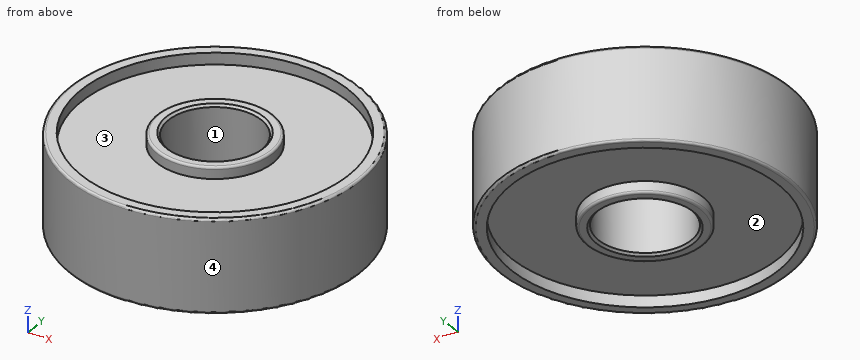
from build123d import *

# Parameters (mm, degrees)
F0_R     = 12.5
F1_DEPTH = 8
F2_R     = 4
F3_DEPTH = 8.001
F2_R_2   = 11.5
F2_R_3   = 5
F4_DEPTH = 1
F5_R     = 11.5
F5_R_2   = 5
F6_DEPTH = 1
F7_R     = 0.2
F8_SIZE  = 0.2


with BuildPart() as f1:
    # F0 (on Top) → F1 (new body)
    with BuildSketch(Plane.XY):
        Circle(F0_R)
    extrude(amount=F1_DEPTH)

    # F2 (on face) → F3 (cut, through all)
    with BuildSketch(Plane.XY.offset(8)):
        Circle(F2_R)
    extrude(amount=-F3_DEPTH, mode=Mode.SUBTRACT)

    # F2 (on face) → F4 (cut)
    with BuildSketch(Plane.XY.offset(8)):
        Circle(F2_R_2)
        Circle(F2_R_3, mode=Mode.SUBTRACT)
    extrude(amount=-F4_DEPTH, mode=Mode.SUBTRACT)

    # F5 (on face) → F6 (cut)
    with BuildSketch(Plane(origin=(0, 0, 0), x_dir=(1, 0, 0), z_dir=(0, 0, -1))):
        Circle(F5_R)
        Circle(F5_R_2, mode=Mode.SUBTRACT)
    extrude(amount=-F6_DEPTH, mode=Mode.SUBTRACT)

    # F7
    f7_edges = [f1.edges().sort_by_distance(p)[0] for p in [
        (-12.5, 0, 8),
        (-12.5, 0, 0),
        (-5, 0, 8),
        (-5, 0, 0),
    ]]
    fillet(f7_edges, radius=F7_R)

    # F8
    f8_edges = [f1.edges().sort_by_distance(p)[0] for p in [
        (-4, 0, 8),
        (-4, 0, 0),
    ]]
    chamfer(f8_edges, length=F8_SIZE)


solid = f1.part
Could you check a few things on this model? Use its own coordinates, in mm. Face numbers are marked on the shaded views. A direction names the side the tool comes from. Coordinates: 2 decimals unless noted, no trailing zeros. Order: outer loops, then holes, each group sorted by start corner. A loop starts at its lowest first (then second) coordinate and runs counter-clockwise, first axis right, second up.
Q1. Please list where these lines run through material, in increasing order: L1, parallel to Y at x = 0, z = 0.75; L2, parallel to Y at x = 0, z = 6.75; L3, parallel to Y at x = -2.25, z = 0.5.
Q2. Will these pins go through, and if not, where does the flat tip stop? pin 1 (8 mm diameter, centred on x = 2.5, y = 4.5, fed in from +Z); pin 2 (2 mm diameter, centred on y = 4, z = 5.5, fed in from -X); pin 3 (1 mm diameter, centred on y = 4, z = 7, fed in from +X); pin 4 (1 mm diameter, centred on x = 3, y = -8.5, fed in from +Z).
Q3. Which directions (+Z, -Z, +X, -X, +Y, -Y) give clear straight access to the entire face, cutting with the end or side of a thin tool? Please do the marked faces 1 and 2.
Q4. Suppose I cut it at A-A on z = 4.25. Please give me the cut outline in (x, y).
Q5. Thinking about a two-plate mould opening in Y: for the marked faces 3 and 4, which applies, released by +Y, released by -Y, zero draft, split by the parting line, or undercut?
Answer:
1. L1: y = -12.5 to -11.5, -5 to -4, 4 to 5, 11.5 to 12.5
1. L2: y = -12.5 to -4, 4 to 12.5
1. L3: y = -12.3 to -11.28, -4.47 to -3.31, 3.31 to 4.47, 11.28 to 12.3
2. pin 1: stops at z = 8
2. pin 2: stops at x = -12.13
2. pin 3: stops at x = 12
2. pin 4: stops at z = 7
3. face 1: +Z, -Z
3. face 2: -Z
4. outline: circle Ø25 at (0, 0); hole circle Ø8 at (0, 0)
5. face 3: undercut
5. face 4: split by the parting line
